Autodesk Inventor part; units mm, degrees
ref_plane "Work Plane2" through (0, 0, 30) normal (0, 0, 1) x (1, 0, 0)
ref_plane "Work Plane3" through (0, 0, -30) normal (0, 0, 1) x (1, 0, 0)
ref_plane "YZ Plane" through (0, 0, 0) normal (1, 0, 0) x (0, 1, 0)
sketch "Sketch1" plane through (0, 0, 0) normal (0, 1, 0) x (-1, 0, 0)
  arc A0 (0, 27) -> (0, -27) centre (0, 0) ccw
  arc A1 (0, 30) -> (0, -30) centre (0, 0) ccw
  line L0 (0, 30) -> (0, 27)
  line L1 (0, -27) -> (0, -30)
  line L2 (0, -30) -> (5, -30)
  line L3 (5, -30) -> (5, -26.533)
  line L4 (5, -26.533) -> (0, -26.533)
  line L5 (0, -26.533) -> (0, -30)
  line L6 (0, 27) -> (5, 27)
  line L7 (5, 27) -> (5, 29.5804)
  line L8 (5, 29.5804) -> (0, 29.5804)
  line L9 (0, 29.5804) -> (0, 27)
  dimension "d0" = 30
  dimension "d1" = 27
  dimension "d31" = 5
  dimension "d32" = 5
extrude "Extrusion1" add sketch "Sketch1" along normal blind 150
ref_plane "Work Plane2" through (0, 0, 30) normal (0, 0, 1) x (1, 0, 0)
sketch "Sketch3" plane through (0, 0, 30) normal (0, 0, 1) x (1, 0, 0)
  circle A0 centre (0, 20) radius 1.5
  circle A1 centre (0, 130) radius 1.5
  line L0 (0, 0) -> (30, 0)
  line L1 (0, 0) -> (0, 150)
  line L2 (30, 150) -> (0, 150)
  line L3 (-5, 0) -> (-5, 150)
  dimension "d14" = 3
  dimension "d15" = 20
  dimension "d17" = 3
  dimension "d18" = 20
  dimension "d33" = 5
  dimension "d34" = 5
extrude "Extrusion3" cut sketch "Sketch3" against normal through all
ref_plane "Work Plane3" through (0, 0, -30) normal (0, 0, 1) x (1, 0, 0)
properties part number "goulotte"
Verification items for the finished model (mm, model axes). A direction names the side the tool comes from. Round coordinates to 2 decimals unless told otherwise and drop trailing zeros. Write each loop counter-clockwise with the first axis right and the second up, starting at its lowest first coordinate (ties: lowest second). Pieces come first, ordered by that corner, then holes.
(1) Section check A-A (x = 10). Enter the section's corners in (y, z).
Returned:
outline: (0, -28.28) - (150, -28.28) - (150, -25.08) - (0, -25.08) - close; (0, 25.08) - (150, 25.08) - (150, 28.28) - (0, 28.28) - close
(2) Access from +Z, -Z, +X, -X, +Y, -Y to the whole of each face (thin tool, end or side, straight path). Record for faces 1 (the flat face through (-3, 74, -26.533)), 2 (the flat face through (-5, 74, -28)).
Returned:
face 1: -X, +Y, -Y
face 2: +Z, -Z, -X, +Y, -Y
(3) Section check B-B (y = 120). Enter the section's corners in (x, z).
Returned:
outline: (-5, -30) - (0, -30) arc R30 ccw to (0, 30) - (0, 29.58) - (-5, 29.58) - (-5, 27) - (0, 27) arc R27 cw to (0, -27) - (0, -26.53) - (-5, -26.53) - close
(4) Material ranges on line 1 (Y direction, x = 0, z = 29); line 2 (Z direction, x = -0.5, y = 46); line 3 (Z direction, x = 12, y = 126), recorded low to high.
Returned:
line 1: y = 0 to 18.5, 21.5 to 128.5, 131.5 to 150
line 2: z = -30 to -26.53, 27 to 29.58
line 3: z = -27.5 to -24.19, 24.19 to 27.5
(5) Depth check by flat-ended pin: pin 1 Ø3 at (x, y) = (20, 30.5) entering from +Z; pin 2 Ø2.5 at (x, y) = (-3, 100.5) entering from +Z; pin 3 Ø0.5 at (y, z) = (137.5, -26.5) entering from +X; pin 4 Ø2.5 at (x, y) = (0, 20) entering from -Z. Enter the tip coordinate at first touch or a pass-through.
Returned:
pin 1: stops at z = 23.62
pin 2: stops at z = 29.58
pin 3: stops at x = 14.52
pin 4: passes through
(6) Mould release check, pull along Z, two halves, no side actions. Record for faces 3 (the flat face through (-3, 74, 29.58)), 4 (the cylindrical face through (26.993, 73.95, -0.594)), 5 (the cylindrical face through (-1.5, 130.07, -28.24)): pulls with the +Z half, pulls with the -Z half, needs draft (parallel to the pull), parting line crosses it, or undercut.
Returned:
face 3: pulls with the +Z half
face 4: undercut
face 5: needs draft
(7) Section check C-C (z = 0). Enter the section's corners in (x, y).
Returned:
outline: (27, 0) - (30, 0) - (30, 150) - (27, 150) - close
